Verification items for the finished model (mm, model axes). Face numbers are marked on the shaded views. A direction names the side the tool comes from. Round coordinates to 2 decimals unless told otherwise and drop trailing zeros. Write each loop counter-clockwise with the first axis right and the second up, starting at its lowest first coordinate (ties: lowest second). Pieces come first, ordered by that corner, then holes. Notation, with made-up numbers: (55, 11.25) - (71, 11.25) arc R19 ccw to (71, 27.25) - close; hole circle Ø10 at (64.5, -13). An arc over 180 degrees is marked (long way). Answer as a JSON object with one key per item and string values.
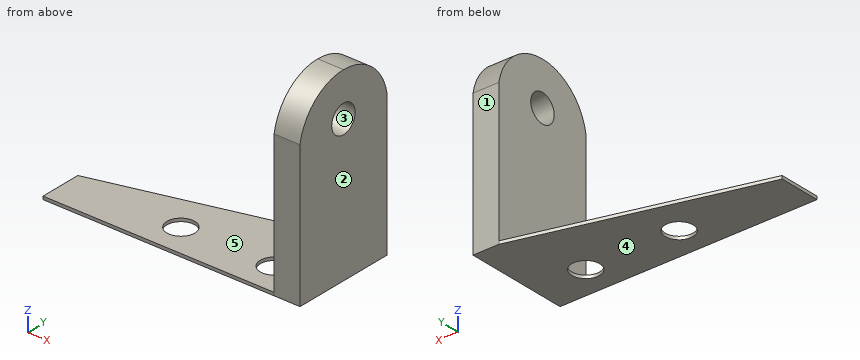
```python
from build123d import *

# Parameters (mm, degrees)
F0_W     = 6.35
F0_H     = 25.4
F1_DEPTH = 45.72
F2_DEPTH = 0.762
F4_DEPTH = 25.4
F3_R     = 3.429
F5_DEPTH = 25.4
F6_R     = 3.429
F7_DEPTH = 25.4


with BuildPart() as f1:
    # F0 (on Top) → F1 (new body)
    with BuildSketch(Plane.XY):
        with Locations((-3.175, -4.690345)):
            Rectangle(F0_W, F0_H)
    extrude(amount=F1_DEPTH)

    # F0 (on Top) → F2 (join)
    with BuildSketch(Plane.XY):
        with Locations((-3.175, -4.690345)):
            Rectangle(F0_W, F0_H)
        Polygon((-62.9412, -17.478447), (-6.35, -17.390345), (-6.35, 8.009655), (-62.9412, -7.318447), align=None)
    extrude(amount=F2_DEPTH)

    # F3 (on face) → F4 (cut)
    with BuildSketch(Plane.YZ):
        with BuildLine():
            ThreePointArc((-4.690345, 45.72), (3.602667, 42.69911), (8.009655, 35.052))
            Line((8.009655, 35.052), (8.009655, 45.72))
            Line((8.009655, 45.72), (-4.690345, 45.72))
        make_face()
        with BuildLine():
            ThreePointArc((-17.390345, 35.052), (-12.983358, 42.69911), (-4.690345, 45.72))
            Line((-4.690345, 45.72), (-17.390345, 45.72))
            Line((-17.390345, 45.72), (-17.390345, 35.052))
        make_face()
    extrude(amount=-F4_DEPTH, mode=Mode.SUBTRACT)

    # F3 (on face) → F5 (cut)
    with BuildSketch(Plane.YZ):
        with Locations((-4.700625, 35.052)):
            Circle(F3_R)
    extrude(amount=-F5_DEPTH, mode=Mode.SUBTRACT)

    # F6 (on face) → F7 (cut)
    with BuildSketch(Plane.XY.offset(0.762)):
        with Locations((-35.56, -9.815811)):
            Circle(F6_R)
        with Locations((-12.7, -9.780222)):
            Circle(F6_R)
    extrude(amount=-F7_DEPTH, mode=Mode.SUBTRACT)


solid = f1.part
```
Q1. Section check B-B, the plane x = -35.56. Record the cut outline in (y, z).
Geometry check:
{"outline": "(-17.44, 0) - (-13.24, 0) - (-13.24, 0.76) - (-17.44, 0.76) - close; (-6.39, 0) - (0.1, 0) - (0.1, 0.76) - (-6.39, 0.76) - close"}
Q2. Gauge pin test, flat ends, axial feed: P1, Ø7, axis at x = -3.5, z = 18, coming from the -Y side; P2, Ø2, axis at y = -8.5, z = 12.5, coming from the -X side; P3, Ø12, axis at x = -50, y = -9.5, coming from the +Z side. Record the tip position at first contact, or that the pin passes through.
Geometry check:
{"P1": "stops at y = -17.39", "P2": "stops at x = -6.35", "P3": "stops at z = 0.76"}
Q3. Section check C-C, the plane z = 37. Record the cut outline in (x, y), then the cut area to 3 significant figures.
Geometry check:
{"outline": "(-6.35, -16.89) - (0, -16.89) - (0, -7.52) - (-6.35, -7.52) - close; (-6.35, -1.88) - (0, -1.88) - (0, 7.51) - (-6.35, 7.51) - close", "area": "119 mm2"}
Q4. Material ranges on line 1 along Z through (x, y) = (-25, -1.75); line 2 along X through (y, z) = (-3.75, 29); line 3 along Y through (x, z) = (-12.7, 0.5), recorded low to high. Write a range as [from, to].
Geometry check:
{"line 1": "z = [0, 0.76]", "line 2": "x = [-6.35, 0]", "line 3": "y = [-17.4, -13.21], [-6.35, 6.29]"}
Q5. Set-up check for the marked faces 4 and 5: record each of +Z, -Z, +X, -X, +Y, -Y from which the full face is reachable in a straight line by a thin tool's end or side.
Geometry check:
{"face 4": "-Z, +X, -X, +Y, -Y", "face 5": "+Z, -X, +Y, -Y"}
Q6. Section check A-A, the plane y = -11.5. Record the cut outline in (x, z), then the cut area to 3 significant figures.
Geometry check:
{"outline": "(-62.94, 0) - (-38.55, 0) - (-38.55, 0.76) - (-62.94, 0.76) - close; (-32.57, 0) - (-15.67, 0) - (-15.67, 0.76) - (-32.57, 0.76) - close; (-9.73, 0) - (0, 0) - (0, 43.78) - (-6.35, 43.78) - (-6.35, 0.76) - (-9.73, 0.76) - close", "area": "312 mm2"}
Q7. Release check for a two-part mould opening along Y. For the marked faces 1, 2 and 3 record: released by +Y, released by -Y, zero draft, split by the parting line, or undercut.
Geometry check:
{"face 1": "released by +Y", "face 2": "zero draft", "face 3": "undercut"}
Q8. Section check D-D, the plane z = 4.5. Record the cut outline in (x, y).
Geometry check:
{"outline": "(-6.35, -17.39) - (0, -17.39) - (0, 8.01) - (-6.35, 8.01) - close"}
